from build123d import *

# Parameters (mm, degrees)
SKETCH1_W           = 396.875
SKETCH1_H           = 238.125
BOSS_EXTRUDE1_DEPTH = 12.7
CUT_EXTRUDE1_DEPTH  = 13.7


with BuildPart() as part:
    # Sketch1 → Boss-Extrude1 (new body)
    with BuildSketch(Plane(origin=(0, 0, 0), x_dir=(1, 0, 0), z_dir=(0, 1, 0))):
        with Locations((198.4375, -119.0625)):
            Rectangle(SKETCH1_W, SKETCH1_H)
    extrude(amount=BOSS_EXTRUDE1_DEPTH)

    # Sketch2 → Cut-Extrude1 (cut, through all)
    with BuildSketch(Plane(origin=(0, 12.7, 0), x_dir=(1, 0, 0), z_dir=(0, 1, 0))):
        Polygon((79.4375, -238.125), (0, -238.125), (0, -195.625), (0, -157.0625), (42.5, -157.0625), (42.5, -195.625), (79.4375, -195.625), align=None)
        Polygon((79.4375, 0), (0, 0), (0, -42.5), (0, -81.0625), (42.5, -81.0625), (42.5, -42.5), (79.4375, -42.5), align=None)
        Polygon((317.4375, 0), (396.875, 0), (396.875, -42.5), (396.875, -81.0625), (354.375, -81.0625), (354.375, -42.5), (317.4375, -42.5), align=None)
        Polygon((317.4375, -238.125), (317.4375, -195.625), (354.375, -195.625), (354.375, -157.0625), (396.875, -157.0625), (396.875, -195.625), (396.875, -238.125), align=None)
    extrude(amount=-CUT_EXTRUDE1_DEPTH, mode=Mode.SUBTRACT)


solid = part.part
Geometry: final body of the model. Coordinates: model frame, mm. A direction names the side the tool comes from. Coordinates: 2 decimals unless noted, no trailing zeros. Order: outer loops, then holes, each group sorted by start corner. A loop starts at its lowest first (then second) coordinate and runs counter-clockwise, first axis right, second up.
(1) Draft query along Y for faces 1 (the face through (196, 0, 117)), 2 (the face through (196, 12.7, 117)), 3 (the face through (354.375, 6, 177)). Return one class per face: pulls with the +Y half, pulls with the -Y half, needs draft (parallel to the pull), parting line crosses it, or undercut.
(2) Section query A-A (y = 2). Return the cut outline in (x, z) (1 decimal).
(3) Section query B-B (x = 66.5). Return the cut outline in (y, z) (3 decimals), plus the area to 3 significant figures.
(4) First-contact query: pin 1 (4 mm diameter, centred on y = 10, z = 192.5, fed in from -X); pin 2 (6.5 mm diameter, centred on x = 68.5, y = 9, fed in from +Z) (3 decimals); pin 3 (4 mm diameter, centred on x = 52, y = 6.5, fed in from -Z). Flat tips, straight axial feed; report the tip coordinate or a pass-through.
(5) Material intervals for probe 1 along Z at (x, y) = (18.5, 0.5); probe 2 along Z at (x, y) = (324, 10.5) (3 decimals); probe 3 along X at (y, z) = (6.75, 74) (3 decimals), sorted ascending.
(6) Access query for faces 4 (the face through (79.438, 6, 217)), 5 (the face through (354.375, 6, 62)), 6 (the face through (336, 6, 195.625)), 7 (the face through (42.5, 6, 62)). Directions: +Z, -Z, +X, -X, +Y, -Y. A direction counts if a zero-diameter tool reaches every point of the face in a straight line with its end or side. Return the directions, or none.
(7) Section query C-C (z = 190). Return the cut outline in (x, y) (3 decimals), plus the area to 3 significant figures.
Solution:
1. face 1: pulls with the -Y half
1. face 2: pulls with the +Y half
1. face 3: needs draft
2. outline: (0, 81.1) - (42.5, 81.1) - (42.5, 42.5) - (79.4, 42.5) - (79.4, 0) - (317.4, 0) - (317.4, 42.5) - (354.4, 42.5) - (354.4, 81.1) - (396.9, 81.1) - (396.9, 157.1) - (354.4, 157.1) - (354.4, 195.6) - (317.4, 195.6) - (317.4, 238.1) - (79.4, 238.1) - (79.4, 195.6) - (42.5, 195.6) - (42.5, 157.1) - (0, 157.1) - close
3. outline: (0, 42.5) - (12.7, 42.5) - (12.7, 195.625) - (0, 195.625) - close
3. area: 1,940 mm2
4. pin 1: stops at x = 42.5
4. pin 2: stops at z = 195.625
4. pin 3: stops at z = 42.5
5. probe 1: z = 81.06 to 157.06
5. probe 2: z = 42.5 to 195.625
5. probe 3: x = 42.5 to 354.375
6. face 4: +Z, -X, +Y, -Y
6. face 5: -Z, +X, +Y, -Y
6. face 6: +Z, +X, +Y, -Y
6. face 7: -Z, -X, +Y, -Y
7. outline: (42.5, 0) - (354.375, 0) - (354.375, 12.7) - (42.5, 12.7) - close
7. area: 3,960 mm2
